Answer from the drawing. Dimensions are ordinates in mm from the lowest x, y and z of the part. A direction names the side the tool comes from. Give positions to 0.01 mm unless a question says otherwise; leave off trailing zeros. Write each loop counter-clockwise with the first axis right and the second up, starting at its lowest first coordinate (ties: lowest second). Pieces come first, ordered by that corner, then holes. Notation, with made-up numbers: (88, 37.25) - (140, 37.25) arc R17 cw to (140, 61.25) - close; hole circle Ø6 at (-11.5, 7). An arc over 180 degrees is marked (long way). Answer as a JSON object with one key per item and string values. Group by question number.
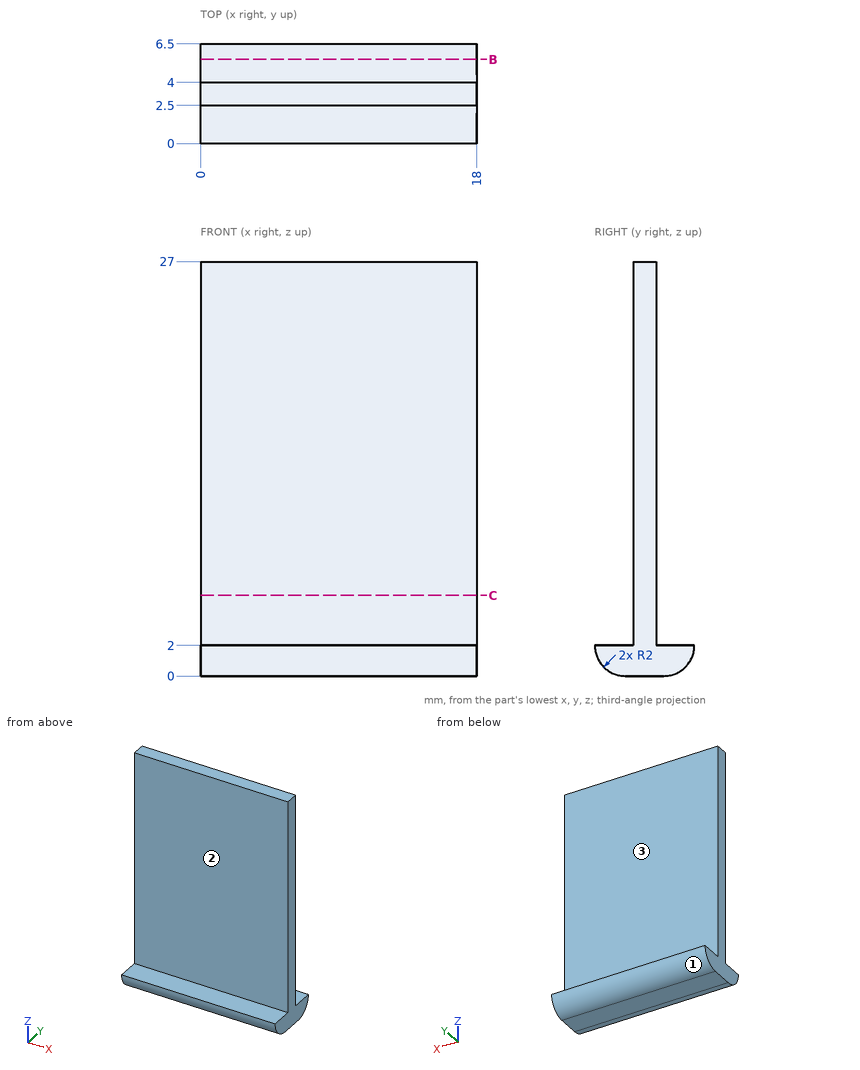
1) Find section B-B, the plane y = 5.5. Write down the section's boundary in (x, z).
2) A flat-ended cylindrical pin translates along its axis: pin 1 Ø1.5 at (x, z) = (2.5, 16.5) entering from +Y. Find the tip coordinate at first contact, or state that the pin passes through.
3) Find section C-C, the plane z = 5.25. Write down the section's boundary in (x, y).
4) Which of the six approach directions +Z, -Z, +X, -X, +Y, -Y give full straight-line access (tool end or side, diameter ignored) to the marked faces 1, 2 and 3?
5) Find the intervals of material crossed by line 1 (Y direction, x = 6.5, z = 8); line 2 (Z direction, x = 13.75, y = 2); line 3 (Z direction, x = 6.5, y = 5.25), in increasing order. Write a range as [from, to].
Values follow:
{
 "1": {"outline": "(0, 0.27) - (18, 0.27) - (18, 2) - (0, 2) - close"},
 "2": {"pin 1": "stops at y = 4"},
 "3": {"outline": "(0, 2.5) - (18, 2.5) - (18, 4) - (0, 4) - close"},
 "4": {"face 1": "-Z, +X, -X, +Y", "face 2": "+Z, +X, -X, -Y", "face 3": "+Z, +X, -X, +Y"},
 "5": {"line 1": "y = [2.5, 4]", "line 2": "z = [0, 2]", "line 3": "z = [0.15, 2]"}
}
